Design review of the part shown in the three views and the two pictorial views. Dimensions are in mm from the part's minimum x, y and z. Give positions to 0.01 mm unless a question says otherwise; leave off trailing zeros. Order: outer loops, then holes, each group sorted by start corner. A loop starts at its lowest first (then second) coordinate and runs counter-clockwise, first axis right, second up.
Item 1: Consider section C-C (z = 1.3). Give the boundary of the cut face in (x, y), plus the area to 3 significant figures.
Item 2: The part is to be moulded in two halves that separate along X. For the marked faces 1, 2, 3 and 4, say which applies: released by +X, released by -X, zero draft, split by the parting line, or undercut.
Item 3: For P1, Ø1, axis at x = 21.5, z = 1.5, coming from the -Y side (3 decimals), flat-tipped, find the tip position at first contact; note if it passes through.
Item 4: Consider section D-D (x = 9.5). Give the boundary of the cut face in (y, z), plus the area to 3 significant figures.
Item 5: For probe 1 along Y at (x, z) = (13.5, 2.2); probe 2 along X at (y, z) = (14, 0.5); probe 3 along X at (y, z) = (12.25, 0.75), list the stretches that pass through material, from the lowest coordinate up.
Item 6: Consider section A-A (y = 13.5). Give the boundary of the cut face in (x, z), plus the area to 3 significant figures.
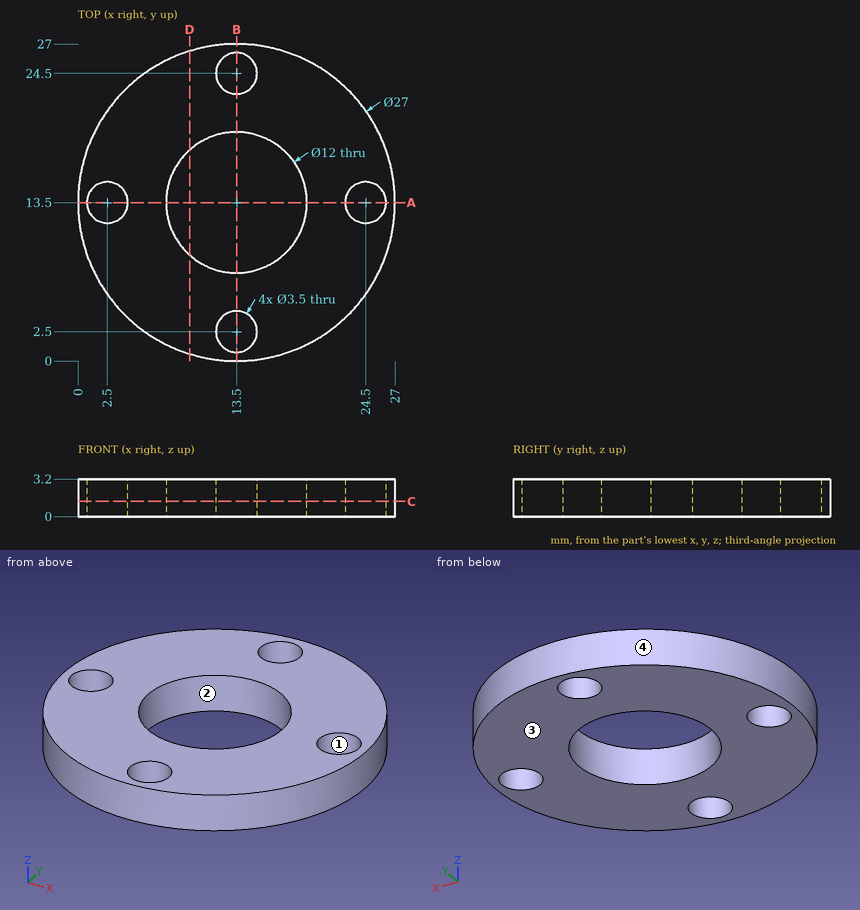
Resolved:
1. outline: circle Ø27 at (13.5, 13.5); hole circle Ø3.5 at (2.5, 13.5); hole circle Ø12 at (13.5, 13.5); hole circle Ø3.5 at (13.5, 2.5); hole circle Ø3.5 at (13.5, 24.5); hole circle Ø3.5 at (24.5, 13.5)
1. area: 421 mm2
2. face 1: undercut
2. face 2: undercut
2. face 3: zero draft
2. face 4: split by the parting line
3. P1: stops at y = 2.275
4. outline: (0.61, 0) - (9.03, 0) - (9.03, 3.2) - (0.61, 3.2) - close; (17.97, 0) - (26.39, 0) - (26.39, 3.2) - (17.97, 3.2) - close
4. area: 53.9 mm2
5. probe 1: y = 0 to 0.75, 4.25 to 7.5, 19.5 to 22.75, 26.25 to 27
5. probe 2: x = 0.01 to 0.82, 4.18 to 7.52, 19.48 to 22.82, 26.18 to 26.99
5. probe 3: x = 0.06 to 1.28, 3.72 to 7.63, 19.37 to 23.28, 25.72 to 26.94
6. outline: (0, 0) - (0.75, 0) - (0.75, 3.2) - (0, 3.2) - close; (4.25, 0) - (7.5, 0) - (7.5, 3.2) - (4.25, 3.2) - close; (19.5, 0) - (22.75, 0) - (22.75, 3.2) - (19.5, 3.2) - close; (26.25, 0) - (27, 0) - (27, 3.2) - (26.25, 3.2) - close
6. area: 25.6 mm2
